Verification items for the finished model (mm, model axes). A direction names the side the tool comes from. Give positions to 0.01 mm unless a question says otherwise; leave off trailing zeros. Loops run counter-clockwise (first coordinate to the right, second up) from the corner with the lowest first, then second, coordinate; pieces in that order, holes last. Notation, with made-up numbers: M -11.75,42 L 43.25,42 A17 cw 43.25,48 Z; hole C -30.5,35.5 d11. An arc over 180 degrees is marked long. Put each result on its own line as item: value. Start each with the question number.
from build123d import *

# Parameters (mm, degrees)
F0_W      = 9.525
F0_H      = 12.7
F1_DEPTH  = 12.7
F2_R      = 3.9751
F3_DEPTH  = 15.875
F4_R      = 3.9751
F5_DEPTH  = 6.35
F6_R      = 1.5875
F7_DEPTH  = 34.926
F8_R      = 1.7272
F9_DEPTH  = 9.526
F10_R     = 2.0828
F11_DEPTH = 8.9916
F12_R     = 0.8001
F13_DEPTH = 6.35


with BuildPart() as f1:
    # F0 (on Front) → F1 (new body)
    with BuildSketch(Plane.XZ):
        with Locations((0.0127, 6.35)):
            Rectangle(F0_W, F0_H)
    extrude(amount=F1_DEPTH)

    # F2 (on face) → F3 (join)
    with BuildSketch(Plane.XZ.offset(12.7)):
        with Locations((0, 7.9248)):
            Circle(F2_R)
    extrude(amount=F3_DEPTH)

    # F4 (on face) → F5 (join)
    with BuildSketch(Plane(origin=(0, 0, 0), x_dir=(-1, 0, 0), z_dir=(0, 1, 0))):
        with Locations((0, 7.9248)):
            Circle(F4_R)
    extrude(amount=F5_DEPTH)

    # F6 (on face) → F7 (cut, through all)
    with BuildSketch(Plane(origin=(0, 6.35, 0), x_dir=(-1, 0, 0), z_dir=(0, 1, 0))):
        with Locations((0, 7.9248)):
            Circle(F6_R)
    extrude(amount=-F7_DEPTH, mode=Mode.SUBTRACT)

    # F8 (on face) → F9 (cut, through all)
    with BuildSketch(Plane.YZ.offset(4.7752)):
        with Locations((-6.35, 5.4356)):
            Circle(F8_R)
    extrude(amount=-F9_DEPTH, mode=Mode.SUBTRACT)

    # F10 (on face) → F11 (cut)
    with BuildSketch(Plane.XY.offset(12.7)):
        with Locations((0, -6.35)):
            Circle(F10_R)
    extrude(amount=-F11_DEPTH, mode=Mode.SUBTRACT)

    # F12 (on face) → F13 (cut)
    with BuildSketch(Plane.XY.offset(12.7)):
        with Locations((3.7338, -11.0236)):
            Circle(F12_R)
    extrude(amount=-F13_DEPTH, mode=Mode.SUBTRACT)

    # F15: sweep along a path in F15_path
    with BuildLine(Plane(origin=(-3.9751, 6.35, 7.9248), x_dir=(0, 0, -1), z_dir=(0, 1, 0))) as f15_path:
        CenterArc((0, -3.9751), 3.9751, 0, 360)
    # F14 (on Right) → F15 (sweep, cut)
    with BuildSketch(Plane.YZ):
        Polygon((6.3891997561, 7.9248), (6.3891997561, 10.8458), (3.8409422638, 9.3745628509), (3.8409422638, 7.9248), align=None)
    sweep(path=f15_path.line, mode=Mode.SUBTRACT)


solid = f1.part
Q1. Release check for a two-part mould opening along Y. For faces 6 (the face through (1.987, -5.724, 9.266)), 7 (the face through (0.2, -0.4, 9.5)), 8 (the face through (-0.1, -12.7, 3.6)) record: pulls with the +Y half, pulls with the -Y half, needs draft (parallel to the pull), parting line crosses it, or undercut.
Q2. Set-up check for faces 1 (the face through (-0.517, -20.526, 11.866)), 2 (the face through (4, -11, 6.35)), 3 (the face through (0.344, -17.99, 6.375)), 4 (the face through (-4.75, -6, 8)), 5 (the face through (-0.1, 0, 3.6)): record each of +Z, -Z, +X, -X, +Y, -Y from which the full face is reachable in a straight line by a thin tool's end or side.
Q3. Cross-section at A-A, the plane x = 0. Record the boundary of the cut face in (y, z) (3 decimals).
Q4. Scan lines: L1, parallel to X at y = -6.5, z = 12; L2, parallel to Z at x = 3.6, y = -6.35; L3, parallel to Y at x = -2.75, z = 5.5 (3 decimals). Record each from-to range of solid material in increasing order.
Q5. Cross-section at C-C, the plane y = -21. Record the boundary of the cut face in (x, z) (1 decimal).
Q6. Cross-section at B-B, the plane z = 2.25. Record the boundary of the cut face in (x, y).
Q7. Go/stop test with flat-tipped pins: pin 1 (1.2 mm diameter, centred on x = 0, y = -6, fed in from +Z); pin 2 (3 mm diameter, centred on x = 1.5, y = -18, fed in from +Z); pin 3 (6 mm diameter, centred on y = -24, z = 11, fed in from +X). Record where each tip stops, or that it passes through.
Ans:
1. face 6: undercut
1. face 7: needs draft
1. face 8: pulls with the -Y half
2. face 1: -Y
2. face 2: +Z
2. face 3: +Y, -Y
2. face 4: +Z, -Z, -X, +Y, -Y
2. face 5: +Y
3. outline: M -28.575,3.95 L -12.7,3.95 L -12.7,0 L 0,0 L 0,3.95 L 6.35,3.95 L 6.35,5.026 L 4.08,6.337 L -4.267,6.337 L -4.267,3.708 L -8.433,3.708 L -8.433,6.337 L -28.575,6.337 Z; M -28.575,9.512 L -8.433,9.512 L -8.433,12.7 L -12.7,12.7 L -12.7,11.9 L -28.575,11.9 Z; M -4.267,9.512 L 4.08,9.512 L 6.35,10.823 L 6.35,11.9 L 0,11.9 L 0,12.7 L -4.267,12.7 Z
4. L1: x = -4.75 to -2.08, 2.08 to 4.78
4. L2: z = 0 to 3.71, 7.16 to 12.7
4. L3: y = -28.575 to -8.076, -4.624 to 6.35
5. outline: C 0,7.9 d8; hole C 0,7.9 d3.2
6. outline: M -4.75,-12.7 L 4.78,-12.7 L 4.78,0 L -4.75,0 Z
7. pin 1: stops at z = 3.71
7. pin 2: stops at z = 11.9
7. pin 3: stops at x = 3.97
